Build history of the part. All positions in model axes, mm. A direction names the side the tool comes from. Round coordinates to 2 decimals unless told otherwise and drop trailing zeros. Order: outer loops, then holes, each group sorted by start corner. A loop starts at its lowest first (then second) coordinate and runs counter-clockwise, first axis right, second up. Notation, with made-up numbers: (-15, 43) -> (-6, 43) arc R17 ccw to (-6, 64) -> close; hole circle Ø8 at (-24, -21). An arc over 180 degrees is marked (long way). Answer as a JSON object with one key per item and string values.
from build123d import *

# Parameters (mm, degrees)
F0_W     = 4.62
F0_H     = 1.02
F0_W_2   = 4.12
F0_H_2   = 0.52
F1_DEPTH = 8
F2_W     = 4.62
F2_H     = 1.02
F3_DEPTH = 1
F5_DEPTH = 4.62


with BuildPart() as f1:
    # F0 (on Right) → F1 (new body)
    with BuildSketch(Plane.YZ):
        with Locations((3.31, 19.710189)):
            Rectangle(F0_W, F0_H)
        with Locations((3.31, 19.710189)):
            Rectangle(F0_W_2, F0_H_2, mode=Mode.SUBTRACT)
    extrude(amount=-F1_DEPTH)

    # F2 (on face) → F3 (join)
    with BuildSketch(Plane.YZ):
        with Locations((3.31, 19.710189)):
            Rectangle(F2_W, F2_H)
    extrude(amount=F3_DEPTH)

    # F4 (on face) → F5 (join)
    with BuildSketch(Plane(origin=(0, 5.62, 0), x_dir=(-1, 0, 0), z_dir=(0, 1, 0))):
        with BuildLine():
            Line((-1, 20.220189), (3.5, 20.220189))
            ThreePointArc((3.5, 20.220189), (1.25, 21.535009), (-1, 20.220189))
        make_face()
    extrude(amount=-F5_DEPTH)


solid = f1.part
1) Cut at B-B, the plane z = 19.75. Give the cut face in (x, y), plus the area to 3 significant figures.
Checked values:
{"outline": "(-8, 1) -> (1, 1) -> (1, 5.62) -> (-8, 5.62) -> (-8, 5.37) -> (0, 5.37) -> (0, 1.25) -> (-8, 1.25) -> close", "area": "8.62 mm²"}
2) Flat gauge pins, fed straight in: pin 1 Ø1.2 at (x, y) = (-3, 3.5) entering from +Z; pin 2 Ø2 at (x, y) = (-7, 4.5) entering from +Z. Where does each tip first touch, or does it go through?
Checked values:
{"pin 1": "stops at z = 21.26", "pin 2": "stops at z = 20.22"}
3) Cut at D-D, the plane x = -0.75. Give the cut face in (y, z).
Checked values:
{"outline": "(1, 19.2) -> (5.62, 19.2) -> (5.62, 21.49) -> (1, 21.49) -> close; hole (1.25, 19.45) -> (5.37, 19.45) -> (5.37, 19.97) -> (1.25, 19.97) -> close"}
4) Cut at C-C, the plane y = 2.8. Give the cut face in (x, z).
Checked values:
{"outline": "(-8, 19.2) -> (1, 19.2) -> (1, 20.22) arc R2.58 ccw to (-3.5, 20.22) -> (-8, 20.22) -> (-8, 19.97) -> (0, 19.97) -> (0, 19.45) -> (-8, 19.45) -> close"}
5) Which spindle directions (+Z, -Z, +X, -X, +Y, -Y) get a long thin tool onto all of the face, cutting with end or side? Do faces 1 (the face through (-4, 3, 19.2)), 2 (the face through (-4, 3, 19.97)), 3 (the face through (-6, 3, 20.22)). Say none if no direction does.
Checked values:
{"face 1": "-Z, +X, -X, +Y, -Y", "face 2": "-X", "face 3": "+Z, -X, +Y, -Y"}
6) Pull direction Y, two halves, no side cores. Call faces 4 (the face through (-4, 3, 19.45)), 5 (the face through (-2, 5.62, 20)), 6 (the face through (-1.288, 3.342, 21.535)): pulls with the +Y half, pulls with the -Y half, needs draft (parallel to the pull), parting line crosses it, or undercut.
Checked values:
{"face 4": "undercut", "face 5": "pulls with the +Y half", "face 6": "needs draft"}
7) Cut at A-A, the plane x = -5.25. Give the cut face in (y, z), plus the area to 3 significant figures.
Checked values:
{"outline": "(1, 19.2) -> (5.62, 19.2) -> (5.62, 20.22) -> (1, 20.22) -> close; hole (1.25, 19.45) -> (5.37, 19.45) -> (5.37, 19.97) -> (1.25, 19.97) -> close", "area": "2.57 mm²"}
8) Probe L1, parallel to Y at x = -1.75, z = 19.9; L2, parallel to Z at x = -5, y = 3.9; L3, parallel to X at y = 3.45, z = 19.5. List the from-to ranges inside material, lowest first. Write a range as from..to.
Checked values:
{"L1": "y = 1..1.25, 5.37..5.62", "L2": "z = 19.2..19.45, 19.97..20.22", "L3": "x = 0..1"}
